from build123d import *

# Parameters (mm, degrees)
SKETCH1_W                    = 412
SKETCH1_H                    = 412
BASE_FLANGE1_DEPTH           = 2
EDGE_FLANGE1_STRIP_W         = 13
EDGE_FLANGE1_STRIP_H         = 2
EDGE_FLANGE1_STRIP_CUT_DEPTH = 412
EDGE_FLANGE1_DEPTH           = 412
EDGE_FLANGE2_STRIP_W         = 13
EDGE_FLANGE2_STRIP_H         = 2
EDGE_FLANGE2_STRIP_CUT_DEPTH = 409.5
EDGE_FLANGE2_DEPTH           = 409.5
EDGE_FLANGE3_STRIP_W         = 13
EDGE_FLANGE3_STRIP_H         = 2
EDGE_FLANGE3_STRIP_CUT_DEPTH = 409.5
EDGE_FLANGE3_DEPTH           = 409.5
EDGE_FLANGE4_STRIP_W         = 13
EDGE_FLANGE4_STRIP_H         = 2
EDGE_FLANGE4_STRIP_CUT_DEPTH = 407
EDGE_FLANGE4_DEPTH           = 407
SKETCH18_R                   = 4
CUT_EXTRUDE1_DEPTH           = 10


# Sheet-metal steps are written as plain solids
with BuildPart() as part:
    # Sketch1 → Base-Flange1 (new body)
    with BuildSketch(Plane.XY):
        with Locations((1, -1)):
            Rectangle(SKETCH1_W, SKETCH1_H)
    extrude(amount=-BASE_FLANGE1_DEPTH)

    # Edge-Flange1 strip (across the edge) → Edge-Flange1 strip cut (cut)
    with BuildSketch(Plane(origin=(207, 205, 0), x_dir=(0, -1, 0), z_dir=(-1, 0, 0))):
        with Locations((-4, -1)):
            Rectangle(EDGE_FLANGE1_STRIP_W, EDGE_FLANGE1_STRIP_H)
    extrude(amount=EDGE_FLANGE1_STRIP_CUT_DEPTH, mode=Mode.SUBTRACT)

    # Edge-Flange1 section (across the edge) → Edge-Flange1 (add)
    with BuildSketch(Plane(origin=(207, 205, 0), x_dir=(0, -1, 0), z_dir=(-1, 0, 0))):
        with BuildLine():
            Line((-2, 2.5), (-2, 18))
            Line((-2, 18), (0, 18))
            Line((0, 18), (0, 2.5))
            ThreePointArc((0, 2.5), (0.732233047, 0.732233047), (2.5, 0))
            Line((2.5, 0), (2.5, -2))
            ThreePointArc((2.5, -2), (-0.681980515, -0.681980515), (-2, 2.5))
        make_face()
    extrude(amount=EDGE_FLANGE1_DEPTH)

    # Edge-Flange2 strip (across the edge) → Edge-Flange2 strip cut (cut)
    with BuildSketch(Plane(origin=(207, -207, 0), x_dir=(-1, 0, 0), z_dir=(0, 1, 0))):
        with Locations((-4, -1)):
            Rectangle(EDGE_FLANGE2_STRIP_W, EDGE_FLANGE2_STRIP_H)
    extrude(amount=EDGE_FLANGE2_STRIP_CUT_DEPTH, mode=Mode.SUBTRACT)

    # Edge-Flange2 section (across the edge) → Edge-Flange2 (add)
    with BuildSketch(Plane(origin=(207, -207, 0), x_dir=(-1, 0, 0), z_dir=(0, 1, 0))):
        with BuildLine():
            Line((-2, 2.5), (-2, 18))
            Line((-2, 18), (0, 18))
            Line((0, 18), (0, 2.5))
            ThreePointArc((0, 2.5), (0.732233047, 0.732233047), (2.5, 0))
            Line((2.5, 0), (2.5, -2))
            ThreePointArc((2.5, -2), (-0.681980515, -0.681980515), (-2, 2.5))
        make_face()
    extrude(amount=EDGE_FLANGE2_DEPTH)

    # Edge-Flange3 strip (across the edge) → Edge-Flange3 strip cut (cut)
    with BuildSketch(Plane(origin=(-205, -207, 0), x_dir=(0, 1, 0), z_dir=(1, 0, 0))):
        with Locations((-4, -1)):
            Rectangle(EDGE_FLANGE3_STRIP_W, EDGE_FLANGE3_STRIP_H)
    extrude(amount=EDGE_FLANGE3_STRIP_CUT_DEPTH, mode=Mode.SUBTRACT)

    # Edge-Flange3 section (across the edge) → Edge-Flange3 (add)
    with BuildSketch(Plane(origin=(-205, -207, 0), x_dir=(0, 1, 0), z_dir=(1, 0, 0))):
        with BuildLine():
            Line((-2, 2.5), (-2, 18))
            Line((-2, 18), (0, 18))
            Line((0, 18), (0, 2.5))
            ThreePointArc((0, 2.5), (0.732233047, 0.732233047), (2.5, 0))
            Line((2.5, 0), (2.5, -2))
            ThreePointArc((2.5, -2), (-0.681980515, -0.681980515), (-2, 2.5))
        make_face()
    extrude(amount=EDGE_FLANGE3_DEPTH)

    # Edge-Flange4 strip (across the edge) → Edge-Flange4 strip cut (cut)
    with BuildSketch(Plane(origin=(-205, 202.5, 0), x_dir=(1, 0, 0), z_dir=(0, -1, 0))):
        with Locations((-4, -1)):
            Rectangle(EDGE_FLANGE4_STRIP_W, EDGE_FLANGE4_STRIP_H)
    extrude(amount=EDGE_FLANGE4_STRIP_CUT_DEPTH, mode=Mode.SUBTRACT)

    # Edge-Flange4 section (across the edge) → Edge-Flange4 (add)
    with BuildSketch(Plane(origin=(-205, 202.5, 0), x_dir=(1, 0, 0), z_dir=(0, -1, 0))):
        with BuildLine():
            Line((-2, 2.5), (-2, 18))
            Line((-2, 18), (0, 18))
            Line((0, 18), (0, 2.5))
            ThreePointArc((0, 2.5), (0.732233047, 0.732233047), (2.5, 0))
            Line((2.5, 0), (2.5, -2))
            ThreePointArc((2.5, -2), (-0.681980515, -0.681980515), (-2, 2.5))
        make_face()
    extrude(amount=EDGE_FLANGE4_DEPTH)

    # Sketch18 → Cut-Extrude1 (cut)
    with BuildSketch(Plane(origin=(0, 0, -2), x_dir=(-1, 0, 0), z_dir=(0, 0, -1))):
        with Locations((-184.5, -184.5)):
            Circle(SKETCH18_R)
        with Locations((182.5, -184.5)):
            Circle(SKETCH18_R)
        with Locations((182.5, 182.5)):
            Circle(SKETCH18_R)
        with Locations((-182.5, 182.5)):
            Circle(SKETCH18_R)
    extrude(amount=-CUT_EXTRUDE1_DEPTH, mode=Mode.SUBTRACT)


solid = part.part
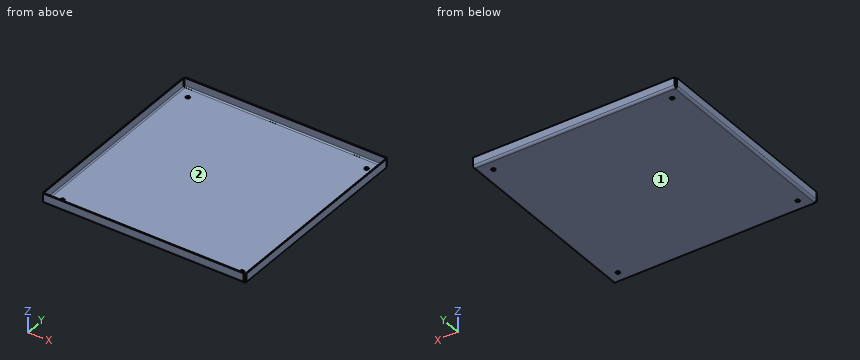
Geometry check sheet. Reference: the model listing, model coordinates, mm. Face numbers are marked on the shaded views. Round coordinates to 2 decimals unless told otherwise and drop trailing zeros. Loops run counter-clockwise (first coordinate to the right, second up) from the corner with the lowest first, then second, coordinate; pieces in that order, holes last. Notation, with made-up numbers: (17.5, 43.25) -> (22.5, 43.25) arc R19 ccw to (22.5, 57.25) -> close; hole circle Ø1 at (-25, 24). An arc over 180 degrees is marked (long way). Answer as a JSON object with one key per item and string values. Group by question number.
Item 1: Cross-section at A-A, the plane z = 14.25. Record the cut outline in (x, y).
Item 2: Release check for a two-part mould opening along Y. For the marked faces 1 and 2 record: pulls with the +Y half, pulls with the -Y half, needs draft (parallel to the pull), parting line crosses it, or undercut.
Item 3: Cross-section at C-C, the plane y = 80.5. Record the cut outline in (x, z).
Item 4: Depth check by flat-ended pin: pin 1 Ø0.6 at (x, z) = (206, -1.5) entering from -Y; pin 2 Ø3 at (x, z) = (-109.5, 0.5) entering from -Y; pin 3 Ø13 at (x, y) = (-182.5, 182.5) entering from -Z; pin 4 Ø5 at (x, y) = (-85.5, -135.5) entering from +Z. Enter the tip coordinate at first touch or a pass-through.
Item 5: Thickness scan on line 1 along Y through (x, z) = (-182.5, -1.25); line 2 along Y through (x, z) = (84, 11); line 3 along X through (y, z) = (151.5, 2). Record the ranges inside material, lowest first.
Item 6: Cross-section at B-B, the plane x = 63. Record the cut outline in (y, z).
Determined:
{
 "1": {"outline": "(-207, -204.5) -> (-205, -204.5) -> (-205, 202.5) -> (-207, 202.5) -> close; (-205, -209) -> (204.5, -209) -> (204.5, -207) -> (-205, -207) -> close; (-205, 205) -> (207, 205) -> (207, 207) -> (-205, 207) -> close; (207, -207) -> (209, -207) -> (209, 202.5) -> (207, 202.5) -> close"},
 "2": {"face 1": "needs draft", "face 2": "undercut"},
 "3": {"outline": "(-207, 2.5) arc R4.5 ccw to (-202.5, -2) -> (204.5, -2) arc R4.5 ccw to (209, 2.5) -> (209, 18) -> (207, 18) -> (207, 2.5) arc R2.5 cw to (204.5, 0) -> (-202.5, 0) arc R2.5 cw to (-205, 2.5) -> (-205, 18) -> (-207, 18) -> close"},
 "4": {"pin 1": "stops at y = -207", "pin 2": "stops at y = -208.97", "pin 3": "stops at z = -2", "pin 4": "stops at z = 0"},
 "5": {"line 1": "y = -206.99 to -188.5, -180.5 to 178.5, 186.5 to 204.99", "line 2": "y = -209 to -207, 205 to 207", "line 3": "x = -206.97 to -204.95, 206.95 to 208.97"},
 "6": {"outline": "(-209, 2.5) arc R4.5 ccw to (-204.5, -2) -> (202.5, -2) arc R4.5 ccw to (207, 2.5) -> (207, 18) -> (205, 18) -> (205, 2.5) arc R2.5 cw to (202.5, 0) -> (-204.5, 0) arc R2.5 cw to (-207, 2.5) -> (-207, 18) -> (-209, 18) -> close"}
}
